from build123d import *

# Parameters (mm, degrees)
BOX004_W      = 10
BOX004_H      = 151
BOX004_DEPTH  = 10
BOX006_W      = 80
BOX006_H      = 10
BOX006_DEPTH  = 10
BOX005_W      = 10
BOX005_H      = 151
BOX005_DEPTH  = 10
BOX007_W      = 80
BOX007_H      = 10
BOX007_DEPTH  = 10
FILLET004_1_R = 2
FILLET004_2_R = 1
BOX003_W      = 116
BOX003_H      = 177
BOX003_DEPTH  = 10
FILLET002_R   = 1.5
BOX002_W      = 120
BOX002_H      = 181
BOX002_DEPTH  = 8
FILLET003_R   = 1.5
BOX001_W      = 98
BOX001_H      = 173.5
BOX001_DEPTH  = 4
FILLET_R      = 1.5
BOX_W         = 120
BOX_H         = 181
BOX_DEPTH     = 4
FILLET001_R   = 1.5


with BuildPart() as cube004:
    # Box004 → Box004 (new body)
    with BuildSketch(Plane(origin=(115, 15, 0), x_dir=(1, 0, 0), z_dir=(0, 0, 1))):
        with Locations((5, 75.5)):
            Rectangle(BOX004_W, BOX004_H)
    extrude(amount=BOX004_DEPTH)


with BuildPart() as cube006:
    # Box006 → Box006 (new body)
    with BuildSketch(Plane(origin=(15, -5, 0), x_dir=(1, 0, 0), z_dir=(0, 0, 1))):
        with Locations((40, 5)):
            Rectangle(BOX006_W, BOX006_H)
    extrude(amount=BOX006_DEPTH)


with BuildPart() as cube005:
    # Box005 → Box005 (new body)
    with BuildSketch(Plane(origin=(0, 15, 0), x_dir=(1, 0, 0), z_dir=(0, 0, 1))):
        with Locations((5, 75.5)):
            Rectangle(BOX005_W, BOX005_H)
    extrude(amount=BOX005_DEPTH)


with BuildPart() as fillet004:
    # Box007 → Box007 (new body)
    with BuildSketch(Plane(origin=(15, 175, 0), x_dir=(1, 0, 0), z_dir=(0, 0, 1))):
        with Locations((40, 5)):
            Rectangle(BOX007_W, BOX007_H)
    extrude(amount=BOX007_DEPTH)

    # Fusion: union Cube004, Cube006, Cube005
    add(cube004.part)
    add(cube006.part)
    add(cube005.part)


with BuildPart() as fillet004_1:
    # Fusion placement: moved
    add(fillet004.part.moved(Location((0, 0, 8))))

    # Fillet004 1
    fillet004_1_edges = [fillet004_1.edges().sort_by_distance(p)[0] for p in [
        (15, 180, 8),
        (95, 180, 8),
        (120, 15, 8),
        (120, 166, 8),
        (95, 0, 8),
        (5, 15, 8),
        (5, 166, 8),
    ]]
    fillet(fillet004_1_edges, radius=FILLET004_1_R)

    # Fillet004 2
    fillet004_2_edges = [fillet004_1.edges().sort_by_distance(p)[0] for p in [
        (15, 0, 8),
    ]]
    fillet(fillet004_2_edges, radius=FILLET004_2_R)


with BuildPart() as fillet002:
    # Box003 → Box003 (new body)
    with BuildSketch(Plane(origin=(4, 2, 4), x_dir=(1, 0, 0), z_dir=(0, 0, 1))):
        with Locations((58, 88.5)):
            Rectangle(BOX003_W, BOX003_H)
    extrude(amount=BOX003_DEPTH)

    # Fillet002
    fillet002_edges = [fillet002.edges().sort_by_distance(p)[0] for p in [
        (4, 2, 9),
        (4, 179, 9),
        (120, 2, 9),
        (120, 179, 9),
    ]]
    fillet(fillet002_edges, radius=FILLET002_R)


with BuildPart() as cut002:
    # Box002 → Box002 (new body)
    with BuildSketch(Plane(origin=(2, 0, 4), x_dir=(1, 0, 0), z_dir=(0, 0, 1))):
        with Locations((60, 90.5)):
            Rectangle(BOX002_W, BOX002_H)
    extrude(amount=BOX002_DEPTH)

    # Fillet003
    fillet003_edges = [cut002.edges().sort_by_distance(p)[0] for p in [
        (2, 0, 8),
        (2, 181, 8),
        (122, 0, 8),
        (122, 181, 8),
    ]]
    fillet(fillet003_edges, radius=FILLET003_R)

    # Cut001: cut Fillet002
    add(fillet002.part, mode=Mode.SUBTRACT)

    # Cut002: cut Fillet004
    add(fillet004_1.part, mode=Mode.SUBTRACT)


with BuildPart() as fillet_body:
    # Box001 → Box001 (new body)
    with BuildSketch(Plane(origin=(7, 4, 0), x_dir=(1, 0, 0), z_dir=(0, 0, 1))):
        with Locations((49, 86.75)):
            Rectangle(BOX001_W, BOX001_H)
    extrude(amount=BOX001_DEPTH)

    # Fillet
    fillet_edges = [fillet_body.edges().sort_by_distance(p)[0] for p in [
        (7, 4, 2),
        (7, 177.5, 2),
        (105, 4, 2),
        (105, 177.5, 2),
    ]]
    fillet(fillet_edges, radius=FILLET_R)


with BuildPart() as fusion001:
    # Box → Box (new body)
    with BuildSketch(Plane(origin=(2, 0, 0), x_dir=(1, 0, 0), z_dir=(0, 0, 1))):
        with Locations((60, 90.5)):
            Rectangle(BOX_W, BOX_H)
    extrude(amount=BOX_DEPTH)

    # Fillet001
    fillet001_edges = [fusion001.edges().sort_by_distance(p)[0] for p in [
        (2, 0, 2),
        (2, 181, 2),
        (122, 0, 2),
        (122, 181, 2),
    ]]
    fillet(fillet001_edges, radius=FILLET001_R)

    # Cut: cut Fillet body
    add(fillet_body.part, mode=Mode.SUBTRACT)

    # Fusion001: union Cut002
    add(cut002.part)


solid = fusion001.part
The listing builds one solid part. Answer for the finished solid, in the listing's coordinates (mm). A direction names the side the tool comes from. Coordinates: 2 decimals unless noted, no trailing zeros. Loops run counter-clockwise (first coordinate to the right, second up) from the corner with the lowest first, then second, coordinate; pieces in that order, holes last. Notation, with made-up numbers: (4.25, 55) -> (35.25, 55) arc R6 ccw to (35.25, 63) -> close; hole circle Ø11 at (28, 12). An arc over 180 degrees is marked (long way). Write item = value, one per line. Start each with the question number.
1) Straight lines are drawn through the part: line 1 (X direction, y = 129, z = 1.5); line 2 (X direction, y = 101.5, z = 6); line 3 (Y direction, x = 97.5, z = 0.75). For each, find the intervals that lie inside material, in ascending order. Write a range as from..to.
2) A cutting plane is placed at A-A (x = 98). Give the vertices of the cut face in (y, z).
3) The mould has two halves that part along Y. Classify faces 4 (the face through (61, 181, 5)), 5 (the face through (106, 118, 0)), 6 (the face through (61, 2, 7)): released by +Y, released by -Y, zero draft, split by the parting line, or undercut.
4) A cutting plane is placed at B-B (y = 143). Give the vertices of the cut face in (x, z).
5) Given pin 1 Ø0.6 at (x, y) = (121.5, 55.5) entering from +Z; pin 2 Ø1.6 at (x, z) = (2.5, 11) entering from -Y; pin 3 Ø5 at (x, y) = (101, 122) entering from +Z, each flat-ended and moving along its own axis, determine where each tip first touches the part or whether it passes through.
6) A tool of negligible diameter and unlimited length cuts with its end or side. For faces 1 (the face through (2, 89, 5)), 2 (the face through (55, 177.5, 2)), 3 (the face through (109, 91, 4)), from which of +Z, -Z, +X, -X, +Y, -Y can it reach the whole face along a straight path? Write none if from no direction.
Responses:
q1.line_1 = 2..7, 105..122
q1.line_2 = 2..4, 120..122
q1.line_3 = 0..4, 177.5..181
q2.outline = (0, 0) -> (4, 0) -> (4, 4) -> (2, 4) -> (2, 12) -> (0, 12) -> close; (177.5, 0) -> (181, 0) -> (181, 12) -> (179, 12) -> (179, 4) -> (177.5, 4) -> close
q3.face_4 = released by +Y
q3.face_5 = zero draft
q3.face_6 = undercut
q4.outline = (2, 0) -> (7, 0) -> (7, 4) -> (4, 4) -> (4, 8) -> (2, 8) -> close; (105, 0) -> (122, 0) -> (122, 8) -> (120, 8) -> (120, 4) -> (105, 4) -> close
q5.pin_1 = 8
q5.pin_2 = 0.01
q5.pin_3 = through
q6.face_1 = +Z, -Z, -X, +Y, -Y
q6.face_2 = +Z, -Z
q6.face_3 = +Z
